For this review, take the finished solid that the model builds, in its own axes (mm). A direction names the side the tool comes from. Round coordinates to 2 decimals unless told otherwise and drop trailing zeros. Order: outer loops, then holes, each group sorted by start corner. A loop starts at its lowest first (then second) coordinate and runs counter-clockwise, first axis right, second up. Notation, with made-up numbers: M 48,12 L 91,12 A18 cw 91,17 Z; hole C 5.25,35.25 d10. An arc over 180 degrees is marked long. Answer in a Markdown table with one row per item. Add a question column.
```python
from build123d import *

# Parameters (mm, degrees)
BASPROSKE_W         = 3
BASPROSKE_H         = 14.625
TOOTHCUT_DEPTH      = 21.89931219
TEETHCUTS_COUNT     = 24
TEETHCUTS_ANGLE     = 345
BORSKE_R            = 1.5
BORE_DEPTH          = 50.0000508
SKETCH1_R           = 1.5
BOSS_EXTRUDE1_DEPTH = 3


with BuildPart() as part:
    # BasProSke → Base-Revolve (revolve)
    with BuildSketch(Plane(origin=(0, 0, 0), x_dir=(1, 0, 0), z_dir=(0, 1, 0)), mode=Mode.PRIVATE) as base_revolve_sk:
        with Locations((1.5, 7.3125)):
            Rectangle(BASPROSKE_W, BASPROSKE_H)
    revolve(base_revolve_sk.sketch.rotate(Axis((-10, 0, 0), (1, 0, 0)), 180), axis=Axis((-10, 0, 0), (1, 0, 0)))

    # TooCutSke → ToothCut (cut, through all)
    with BuildSketch(Plane(origin=(0, 0, 0), x_dir=(0, 0, -1), z_dir=(1, 0, 0))):
        with BuildLine():
            ThreePointArc((0.542722358, 12.080565177), (0, 12.09275), (-0.542722358, 12.080565177))
            ThreePointArc((-0.542722358, 12.080565177), (-0.922320579, 13.38903626), (-1.617327261, 14.56085412))
            ThreePointArc((-1.617327261, 14.56085412), (0, 14.6504), (1.617327261, 14.56085412))
            ThreePointArc((1.617327261, 14.56085412), (0.922320579, 13.38903626), (0.542722358, 12.080565177))
        make_face()
    toothcut = extrude(amount=TOOTHCUT_DEPTH, mode=Mode.SUBTRACT)

    # TeethCuts: ToothCut ×24 about axis
    teethcuts_axis = Axis((-10, 0, 0), (1, 0, 0))
    for i in range(1, TEETHCUTS_COUNT):
        add(toothcut.rotate(teethcuts_axis, i * TEETHCUTS_ANGLE / (TEETHCUTS_COUNT - 1)), mode=Mode.SUBTRACT)

    # BorSke → Bore (cut, symmetric)
    with BuildSketch(Plane(origin=(0, 0, 0), x_dir=(0, 0, -1), z_dir=(1, 0, 0))):
        with Locations(Location((0, 0, 0), (0, 0, 180))):
            Circle(BORSKE_R)
    extrude(amount=BORE_DEPTH, both=True, mode=Mode.SUBTRACT)

    # Sketch1 → Boss-Extrude1 (add)
    with BuildSketch(Plane(origin=(0, 0, 0), x_dir=(0, 0, -1), z_dir=(1, 0, 0))):
        with BuildLine():
            Line((31, 3.650909885), (11.528463019, 3.650909885))
            Line((11.528463019, 3.650909885), (11.528463019, -3.650909885))
            Line((11.528463019, -3.650909885), (31, -3.650909885))
            ThreePointArc((31, -3.650909885), (34.650909885, 0), (31, 3.650909885))
        make_face()
        with Locations((31, 0)):
            Circle(SKETCH1_R, mode=Mode.SUBTRACT)
    extrude(amount=BOSS_EXTRUDE1_DEPTH)


solid = part.part
```
1. To check wall thickness, follow probe 1 along Y at (x, z) = (1, 0); probe 2 along Z at (x, y) = (0.25, -1); probe 3 along Z at (x, y) = (1.9, 12.75). State the ranges of each line that lie inside material, in increasing order. Write a range as [from, to].
2. Consider section D-D on y = 4.25. Write out the cut boundary in (x, z), plus the area to 3 significant figures.
3. Consider section B-B on z = -12.5. Write out the cut boundary in (x, y), plus the area to 3 significant figures.
4. Consider section A-A on y = 0. Write out the cut boundary in (x, z), plus the area to 3 significant figures.
5. Clearance check with flat-ended pins moving along their axes: pin 1 Ø2.5 at (y, z) = (0, 0) entering from +X; pin 2 Ø1.5 at (x, z) = (2.5, -21) entering from -Y. State where each tip first meets the part, or that it passes through.
6. Consider section C-C on x = 0.9. State how many separate pieces and enclosed holes the cut face has, plus the area to 3 significant figures.
7. The part is to be moulded in two halves that separate along Z. For faces 1 (the cylindrical face through (1.48, -0.91, 13.36)), 2 (the cylindrical face through (1.48, -0.08, -34.65)), 3 (the cylindrical face through (1.479, 12.668, 4.335)), say which applies: pulls with the +Z half, pulls with the -Z half, needs draft (parallel to the pull), parting line crosses it, or undercut.
8. For faces 4 (the cylindrical face through (1.479, -13.393, 0.924)), 5 (the cylindrical face through (1.479, -2.574, 13.176)), 6 (the cylindrical face through (1.48, 12.7, -4.36)), list the 3-axis set-ups (+Z, -Z, +X, -X, +Y, -Y) from which the entire face can be reached by the end or side of a thin tool; tool diameter is ignored.
Solved:
| question | item | result |
|---|---|---|
| 1 | probe 1 | y = [-12.09, -1.5], [1.5, 12.09] |
| 1 | probe 2 | z = [-34.51, -32.12], [-29.88, -1.12], [1.12, 13.56] |
| 1 | probe 3 | z = [-5.93, -4.4], [-2.62, -0.69], [0.69, 2.62], [4.4, 5.93] |
| 2 | outline | M 0,-12.56 L 3,-12.56 L 3,12.56 L 0,12.56 Z |
| 2 | area | 75.3 mm^2 |
| 3 | outline | M 0,-5.93 L 3,-5.93 L 3,-4.21 L 0,-4.21 Z; M 0,-3.65 L 3,-3.65 L 3,3.65 L 0,3.65 Z; M 0,4.21 L 3,4.21 L 3,5.93 L 0,5.93 Z |
| 3 | area | 32.2 mm^2 |
| 4 | outline | M 0,-34.65 L 3,-34.65 L 3,-32.5 L 0,-32.5 Z; M 0,-29.5 L 3,-29.5 L 3,-1.5 L 0,-1.5 Z; M 0,1.5 L 3,1.5 L 3,12.09 L 0,12.09 Z |
| 4 | area | 122 mm^2 |
| 5 | pin 1 | passes through |
| 5 | pin 2 | stops at y = -3.65 |
| 6 | separate pieces | 1 |
| 6 | enclosed holes | 2 |
| 6 | area | 694 mm^2 |
| 7 | face 1 | pulls with the +Z half |
| 7 | face 2 | pulls with the -Z half |
| 7 | face 3 | undercut |
| 8 | face 4 | +X, -X, -Y |
| 8 | face 5 | +X, -X |
| 8 | face 6 | +X, -X, +Y |
